from build123d import *

# Parameters (mm, degrees)
SKETCH_1_W          = 40
SKETCH_1_H          = 15
SKETCH_1_R          = 3
EXTRUDE_1_DEPTH     = 10
EXTRUDE_2_DEPTH     = 10
FILLET_1_R          = 1.5
SKETCH_5_R          = 3.5
CUT_EXTRUDE_1_DEPTH = 13
SKETCH_6_R          = 1.75
CUT_EXTRUDE_2_DEPTH = 13
CUT_EXTRUDE_3_DEPTH = 13
FILLET_2_R          = 1


with BuildPart() as part:
    # 草图1 → 凸台-拉伸1 (new body)
    with BuildSketch(Plane.XY):
        with Locations((0, 7.5)):
            Rectangle(SKETCH_1_W, SKETCH_1_H)
        with Locations((-10, 9)):
            Circle(SKETCH_1_R, mode=Mode.SUBTRACT)
        with Locations((10, 9)):
            Circle(SKETCH_1_R, mode=Mode.SUBTRACT)
    extrude(amount=EXTRUDE_1_DEPTH)

    # 草图4 → 凸台-拉伸2 (add)
    with BuildSketch(Plane.XY.offset(10)):
        Polygon((-6.9, -1.8), (-6.9, 0), (-13.1, 0), (-13.1, -1.8), (-15.5, -1.8), (-15.5, -3.439339828), (-12.839339828, -6.1), (-7.160660172, -6.1), (-4.5, -3.439339828), (-4.5, -1.8), align=None)
        Polygon((13.1, -1.8), (13.1, 0), (6.9, 0), (6.9, -1.8), (4.5, -1.8), (4.5, -3.439339828), (7.160660172, -6.1), (12.839339828, -6.1), (15.5, -3.439339828), (15.5, -1.8), align=None)
    extrude(amount=-EXTRUDE_2_DEPTH)

    # 圆角1
    fillet_1_edges = [part.edges().sort_by_distance(p)[0] for p in [
        (20, 15, 5),
        (-20, 15, 5),
    ]]
    fillet(fillet_1_edges, radius=FILLET_1_R)

    # 草图5 → 切除-拉伸1 (cut)
    with BuildSketch(Plane(origin=(0, 15, 0), x_dir=(1, 0, 0), z_dir=(0, 1, 0))):
        with Locations(Location((-10, -5, 0), (0, 0, 270))):
            Circle(SKETCH_5_R)
        with Locations(Location((10, -5, 0), (0, 0, 270))):
            Circle(SKETCH_5_R)
    extrude(amount=-CUT_EXTRUDE_1_DEPTH, mode=Mode.SUBTRACT)

    # 草图6 → 切除-拉伸2 (cut)
    with BuildSketch(Plane(origin=(0, 2, 0), x_dir=(1, 0, 0), z_dir=(0, 1, 0))):
        with Locations(Location((10, -5, 0), (0, 0, 270))):
            Circle(SKETCH_6_R)
        with Locations(Location((-10, -5, 0), (0, 0, 270))):
            Circle(SKETCH_6_R)
    extrude(amount=-CUT_EXTRUDE_2_DEPTH, mode=Mode.SUBTRACT)

    # 草图7 → 切除-拉伸3 (cut)
    with BuildSketch(Plane.XY.offset(10)):
        Polygon((0, 4), (-4, 4), (-4, 0), (4, 0), (4, 4), align=None)
    extrude(amount=-CUT_EXTRUDE_3_DEPTH, mode=Mode.SUBTRACT)

    # 圆角2
    fillet_2_edges = [part.edges().sort_by_distance(p)[0] for p in [
        (4, 4, 5),
        (4, 0, 5),
        (-4, 0, 5),
        (-4, 4, 5),
    ]]
    fillet(fillet_2_edges, radius=FILLET_2_R)


solid = part.part
Could you check a few things on this model? Use its own coordinates, in mm. A direction names the side the tool comes from. Give positions to 0.01 mm unless a question says otherwise; leave off trailing zeros. Order: outer loops, then holes, each group sorted by start corner. A loop starts at its lowest first (then second) coordinate and runs counter-clockwise, first axis right, second up. Notation, with made-up numbers: (46.5, 47.5) -> (64.5, 47.5) arc R16 cw to (64.5, 65.5) -> close; hole circle Ø8 at (18, 11.25). An arc over 180 degrees is marked (long way). Return JSON: item names as keys, results as strings.
1. Imagine slicing it at A-A on x = -10. List the corners of the cut face in (y, z) for me.
Answer list:
{"outline": "(-6.1, 0) -> (6, 0) -> (6, 1.5) -> (2, 1.5) -> (2, 3.25) -> (-6.1, 3.25) -> close; (-6.1, 6.75) -> (2, 6.75) -> (2, 8.5) -> (6, 8.5) -> (6, 10) -> (-6.1, 10) -> close; (12, 0) -> (15, 0) -> (15, 1.5) -> (12, 1.5) -> close; (12, 8.5) -> (15, 8.5) -> (15, 10) -> (12, 10) -> close"}
2. I need wall thicknesses on line 1 (X direction, y = 9, z = 2.1); line 2 (X direction, y = 11.25, z = 5); line 3 (X direction, y = -0.5, z = 5.75). Which ranges of each line are inside material? Lowest first, please. Write a range as from..to.
Answer list:
{"line 1": "x = -20..-13, -7..7, 13..20", "line 2": "x = -20..-13.5, -6.5..6.5, 13.5..20", "line 3": "x = -13.1..-11.58, -8.42..-6.9, 6.9..8.42, 11.58..13.1"}
3. On a 3-axis mill with a long thin cutter (end or side, diameter ignored), from which of +Z, -Z, +X, -X, +Y, -Y can I reach the whole of each face in a straight line? I mean faces 1 (the flat face through (6, -1.8, 5)), 2 (the flat face through (4, 2, 5)), 3 (the cylindrical face through (-13.417, 8.591, 4.241)), 4 (the flat face through (15.5, -3, 5)). Say none if no direction works.
Answer list:
{"face 1": "+Z, -Z", "face 2": "+Z, -Z, -Y", "face 3": "+Y", "face 4": "+Z, -Z, +X, -Y"}
4. Imagine slicing it at D-D on y = 5. List the corners of the cut face in (x, z) for me, then the cut area to 3 significant figures.
Answer list:
{"outline": "(-20, 0) -> (20, 0) -> (20, 10) -> (-20, 10) -> close; hole circle Ø7 at (-10, 5); hole circle Ø7 at (10, 5)", "area": "323 mm2"}
5. Thinking about a two-plate mould opening in Y: for faces 5 (the cylindrical face through (3.715, 3.699, 4.93)), 6 (the flat face through (-8, 2, 6)), 7 (the cylindrical face through (-13, 9, 1)), which applies, pulls with the +Y half, pulls with the -Y half, needs draft (parallel to the pull), parting line crosses it, or undercut?
Answer list:
{"face 5": "pulls with the -Y half", "face 6": "pulls with the +Y half", "face 7": "undercut"}
6. Imagine slicing it at B-B on y = 9. List the corners of the cut face in (x, z) for me, then the cut area to 3 significant figures.
Answer list:
{"outline": "(-20, 0) -> (-13, 0) -> (-13, 3.2) arc R3.5 cw to (-13, 6.8) -> (-13, 10) -> (-20, 10) -> close; (-7, 0) -> (7, 0) -> (7, 3.2) arc R3.5 cw to (7, 6.8) -> (7, 10) -> (-7, 10) -> (-7, 6.8) arc R3.5 cw to (-7, 3.2) -> close; (13, 0) -> (20, 0) -> (20, 10) -> (13, 10) -> (13, 6.8) arc R3.5 cw to (13, 3.2) -> close", "area": "275 mm2"}
7. For pin 1 Ø0.5 at (y, z) = (-1.5, 5.5) entering from +X; pin 2 Ø1.4 at (y, z) = (-1, 5.5) entering from -X; pin 3 Ø0.5 at (y, z) = (-2.5, 7) entering from -X, each with a flat end and sliding along its axis, tell me the tip position at first contact or that it passes through.
Answer list:
{"pin 1": "stops at x = 13.1", "pin 2": "stops at x = -13.1", "pin 3": "stops at x = -15.5"}
8. Imagine slicing it at C-C on x = -6. List the corners of the cut face in (y, z) for me, then the cut area to 3 significant figures.
Answer list:
{"outline": "(-4.94, 0) -> (-1.8, 0) -> (-1.8, 10) -> (-4.94, 10) -> close; (0, 0) -> (15, 0) -> (15, 10) -> (0, 10) -> close", "area": "181 mm2"}
